Verification items for this drawing (mm, ordinates from the low corner). A direction names the side the tool comes from. Round coordinates to 2 decimals unless told otherwise and drop trailing zeros. Loops run counter-clockwise (first coordinate to the right, second up) from the corner with the lowest first, then second, coordinate; pieces in that order, holes last. Notation, with made-up numbers: (-0.75, 74) -> (12.25, 74) arc R21 ccw to (12.25, 91) -> close; hole circle Ø9 at (41, 37). An arc over 180 degrees is marked (long way). One line per item, written item: value. Start each with the question number.
1. Cross-section at B-B on x = 22. Record the cut outline in (y, z).
2. Material ranges on L1, parallel to X at y = 12.25, z = 11.5; L2, parallel to X at y = 19.5, z = 10; L3, parallel to X at y = 13.5, z = 31.5, recorded low to high.
3. Cross-section at A-A on y = 7.25. Record the cut outline in (x, z), then the cut area to 3 significant figures.
4. Go/stop test with flat-tipped pins: pin 1 (1.5 mm diameter, centred on x = 36.5, y = 12.5, fed in from -Z); pin 2 (10 mm diameter, centred on x = 12.5, y = 11.5, fed in from -Z); pin 3 (7.5 mm diameter, centred on x = 24.5, y = 14, fed in from -Z). Record where each tip stops, or that it passes through.
5. Release check for a two-part mould opening along X. For the marked faces 1, 2, 3 and 4 record: +X half, -X half, draft (parallel to the pull), parting line (faces both ways), or undercut.
6. Set-up check for the marked faces 5, 6 and 7: record each of +Z, -Z, +X, -X, +Y, -Y from which the full face is reachable in a straight line by a thin tool's end or side.
7. Cross-section at C-C on z = 33. Record the cut outline in (x, y).
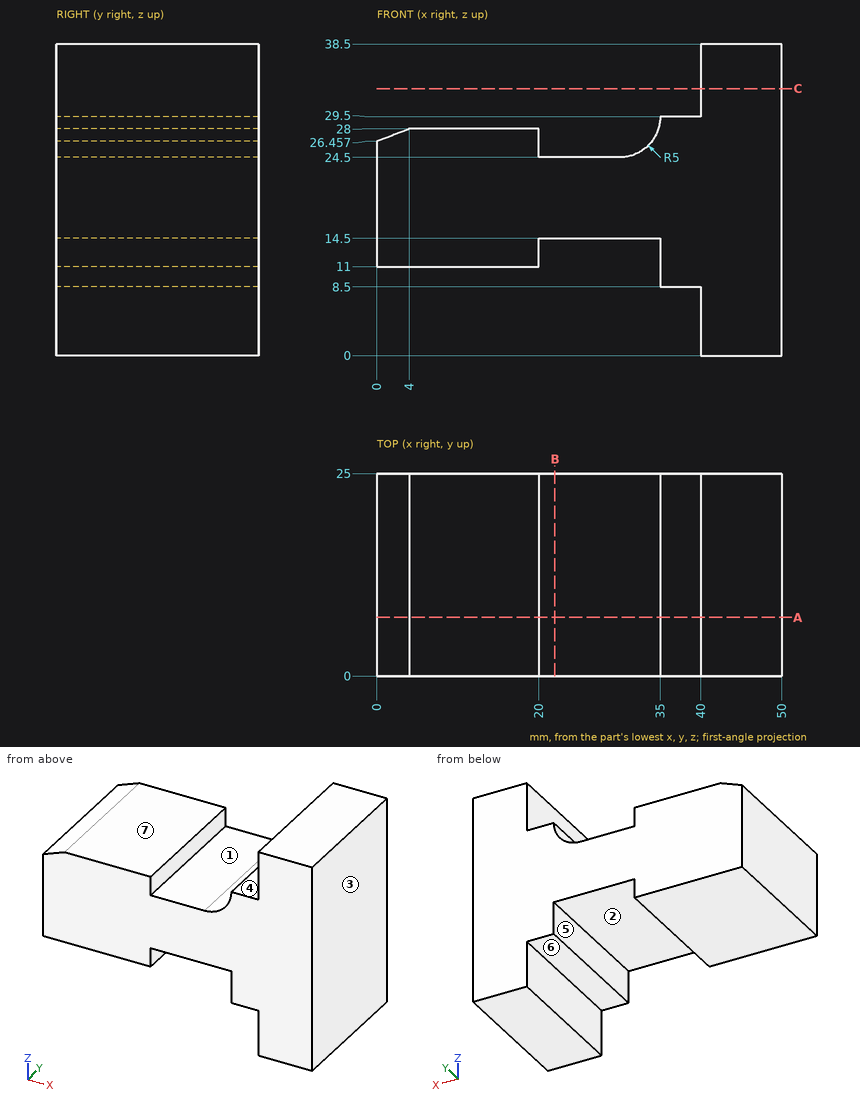
Taken from the geometry:
1. outline: (0, 14.5) -> (25, 14.5) -> (25, 24.5) -> (0, 24.5) -> close
2. L1: x = 0 to 20, 35 to 50
2. L2: x = 35 to 50
2. L3: x = 40 to 50
3. outline: (0, 11) -> (20, 11) -> (20, 14.5) -> (35, 14.5) -> (35, 8.5) -> (40, 8.5) -> (40, 0) -> (50, 0) -> (50, 38.5) -> (40, 38.5) -> (40, 29.5) -> (35, 29.5) arc R5 cw to (30, 24.5) -> (20, 24.5) -> (20, 28) -> (4, 28) -> (0, 26.46) -> close
3. area: 982 mm2
4. pin 1: stops at z = 8.5
4. pin 2: stops at z = 11
4. pin 3: stops at z = 14.5
5. face 1: undercut
5. face 2: undercut
5. face 3: +X half
5. face 4: draft
6. face 5: -Z, +Y, -Y
6. face 6: -Z, -X, +Y, -Y
6. face 7: +Z, -X, +Y, -Y
7. outline: (40, 0) -> (50, 0) -> (50, 25) -> (40, 25) -> close
